Geometry: final body of the model. Coordinates: model frame, mm. A direction names the side the tool comes from. Give positions to 0.01 mm unless a question says otherwise; leave off trailing zeros. Order: outer loops, then holes, each group sorted by start corner. A loop starts at its lowest first (then second) coordinate and runs counter-clockwise, first axis right, second up. Notation, with made-up numbers: (13.5, 61.25) -> (22.5, 61.25) arc R8 cw to (22.5, 74.25) -> close; hole circle Ø2 at (62.25, 87). An arc over 180 degrees is marked (long way). One line per item, written item: value. Start each with the question number.
```python
from build123d import *

# Parameters (mm, degrees)
EXTRUDE_1_DEPTH     = 41.402
SKETCH_4_R          = 7.112
CUT_EXTRUDE_1_DEPTH = 83.979969858
SKETCH_3_R          = 7.112
CUT_EXTRUDE_2_DEPTH = 83.979969858
SKETCH1_R           = 3.175
CUT_EXTRUDE1_DEPTH  = 83.979969858


with BuildPart() as part:
    # 草图1 → 凸台-拉伸1 (new body)
    with BuildSketch(Plane.XY):
        with BuildLine():
            Line((2.54, 0), (50.8, 0))
            Line((50.8, 0), (50.8, 6.35))
            Line((50.8, 6.35), (8.89, 6.35))
            ThreePointArc((8.89, 6.35), (7.093948776, 7.093948776), (6.35, 8.89))
            Line((6.35, 8.89), (6.35, 50.900980282))
            Line((6.35, 50.900980282), (0, 50.900980282))
            Line((0, 50.900980282), (0, 2.54))
            ThreePointArc((0, 2.54), (0.743948776, 0.743948776), (2.54, 0))
        make_face()
    extrude(amount=EXTRUDE_1_DEPTH)

    # 草图4 → 切除-拉伸1 (cut, through all)
    with BuildSketch(Plane.ZY):
        with Locations((20.701, 28.448)):
            Circle(SKETCH_4_R)
    extrude(amount=-CUT_EXTRUDE_1_DEPTH, mode=Mode.SUBTRACT)

    # 草图3 → 切除-拉伸2 (cut, through all)
    with BuildSketch(Plane(origin=(0, 0, 0), x_dir=(-1, 0, 0), z_dir=(0, -1, 0))):
        with Locations(Location((-31.75, -20.701, 0), (0, 0, 90))):
            Circle(SKETCH_3_R)
    extrude(amount=-CUT_EXTRUDE_2_DEPTH, mode=Mode.SUBTRACT)

    # Sketch1 → Cut-Extrude1 (cut, through all)
    with BuildSketch(Plane(origin=(0, 0, 0), x_dir=(-1, 0, 0), z_dir=(0, -1, 0))):
        with Locations(Location((-43.18, -10.38225, 0), (0, 0, 90))):
            Circle(SKETCH1_R)
        with Locations(Location((-43.18, -31.01975, 0), (0, 0, 90))):
            Circle(SKETCH1_R)
    extrude(amount=-CUT_EXTRUDE1_DEPTH, mode=Mode.SUBTRACT)


solid = part.part
```
1. Cut plane C-C, the plane z = 22. Return loops of the section in (x, y).
2. Cut plane D-D, the plane x = 43.18. Return loops of the section in (y, z).
3. Cut plane A-A, the plane x = 31.75. Return loops of the section in (y, z), then the cut area to 3 significant figures.
4. Material intervals for L1, parallel to Y at x = 20, z = 16; L2, parallel to Z at x = 2, y = 22, sorted ascending. Write a range as [from, to].
5. Access query for faces 4 (the flat face through (25, 6.35, 16)), 5 (the cylindrical face through (40.08, 3.13, 11.07)). Directions: +Z, -Z, +X, -X, +Y, -Y. A direction counts if a zero-diameter tool reaches every point of the face in a straight line with its end or side. Return the directions, or none.
6. Draft query along X for faces 1 (the cylindrical face through (3.1, 33.3, 15.5)), 2 (the cylindrical face through (25.44, 3.13, 17.42)), 3 (the flat face through (0, 22, 25)). Return one class per face: pulls with the +X half, pulls with the -X half, needs draft (parallel to the pull), parting line crosses it, or undercut.
7. Pin query (flat end, axial travel): P1, Ø2, axis at y = 25, z = 12.5, coming from the +X side; P2, Ø8, axis at x = 42.5, z = 6.5, coming from the +Y side; P3, Ø13, axis at x = 31.75, z = 20.701, coming from the -Y side. Return the tip coordinate at first contact, or that it passes through.
8. Cut plane B-B, the plane y = 4.5. Return loops of the section in (x, z) (3 decimals), then the cut area to 3 significant figures.
Answers follow:
1. outline: (0, 2.54) arc R2.54 ccw to (2.54, 0) -> (24.76, 0) -> (24.76, 6.35) -> (8.89, 6.35) arc R2.54 cw to (6.35, 8.89) -> (6.35, 21.46) -> (0, 21.46) -> close; (0, 35.44) -> (6.35, 35.44) -> (6.35, 50.9) -> (0, 50.9) -> close; (38.74, 0) -> (50.8, 0) -> (50.8, 6.35) -> (38.74, 6.35) -> close
2. outline: (0, 0) -> (6.35, 0) -> (6.35, 7.21) -> (0, 7.21) -> close; (0, 13.56) -> (6.35, 13.56) -> (6.35, 27.84) -> (0, 27.84) -> close; (0, 34.19) -> (6.35, 34.19) -> (6.35, 41.4) -> (0, 41.4) -> close
3. outline: (0, 0) -> (6.35, 0) -> (6.35, 13.59) -> (0, 13.59) -> close; (0, 27.81) -> (6.35, 27.81) -> (6.35, 41.4) -> (0, 41.4) -> close
3. area: 173 mm²
4. L1: y = [0, 6.35]
4. L2: z = [0, 17.7], [23.7, 41.4]
5. face 4: +Z, -Z, +X, +Y
5. face 5: +Y, -Y
6. face 1: needs draft
6. face 2: undercut
6. face 3: pulls with the -X half
7. P1: stops at x = 6.35
7. P2: stops at y = 6.35
7. P3: passes through
8. outline: (0, 0) -> (50.8, 0) -> (50.8, 41.402) -> (0, 41.402) -> close; hole circle Ø14.224 at (31.75, 20.701); hole circle Ø6.35 at (43.18, 10.382); hole circle Ø6.35 at (43.18, 31.02)
8. area: 1,880 mm²
